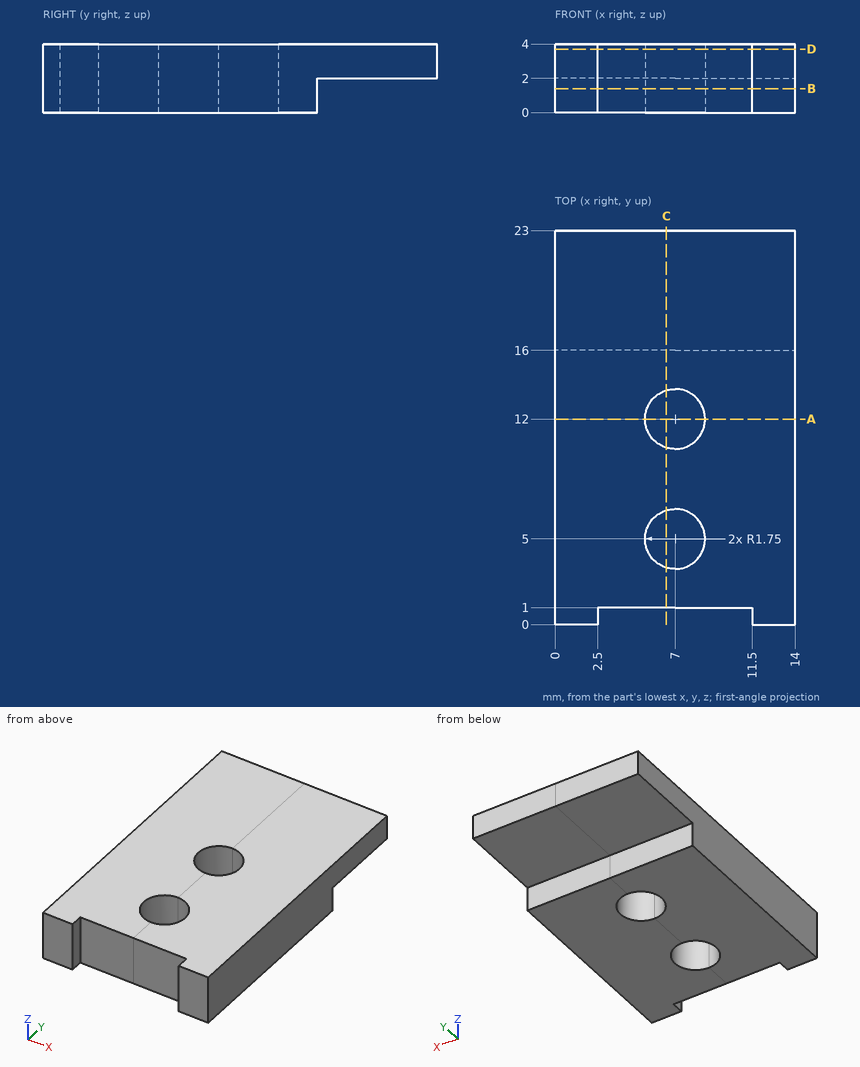
Here's the drawing with two shaded views (mm, measured from the low corner). I have some questions. Give positions to 0.01 mm unless a question says otherwise; leave off trailing zeros. Order: outer loops, then holes, each group sorted by start corner. A loop starts at its lowest first (then second) coordinate and runs counter-clockwise, first axis right, second up.
Q1. If I drill on line 1 along X through (y, z) = (12, 2.85); line 2 along Y through (x, z) = (6.75, 1.55); line 3 along Y through (x, z) = (8.25, 1.4), over which ranges is the centre line in solid material (lowest first)?
Q2. I'm going to push flat-ended pins straight in: P1, Ø4, axis at x = 5, y = 16.5, coming from the -Z side; P2, Ø1.2, axis at x = 9.5, z = 3, coming from the -Y side; P3, Ø0.6, axis at x = 4, z = 1, coming from the +Y side; P4, Ø5.5, axis at x = 9.5, y = 19, coming from the -Z side. Where does each tip first touch, or does it pass through?
Q3. Suppose I cut it at A-A, the plane y = 12. Write out the boundary of the cut face in (x, z), and give its area (3 significant figures).
Q4. Suppose I cut it at B-B, the plane z = 1.4. Write out the boundary of the cut face in (x, y).
Q5. Suppose I cut it at D-D, the plane z = 3.7. Write out the boundary of the cut face in (x, y).
Q6. Suppose I cut it at C-C, the plane x = 6.5. Write out the boundary of the cut face in (y, z), and give its area (3 significant figures).
Solution:
1. line 1: x = 0 to 5.25, 8.75 to 14
1. line 2: y = 1 to 3.27, 6.73 to 10.27, 13.73 to 16
1. line 3: y = 1 to 3.78, 6.22 to 10.78, 13.22 to 16
2. P1: stops at z = 0
2. P2: stops at y = 1
2. P3: stops at y = 16
2. P4: stops at z = 2
3. outline: (0, 0) - (5.25, 0) - (5.25, 4) - (0, 4) - close; (8.75, 0) - (14, 0) - (14, 4) - (8.75, 4) - close
3. area: 42.0 mm2
4. outline: (0, 0) - (2.5, 0) - (2.5, 1) - (11.5, 1) - (11.5, 0) - (14, 0) - (14, 16) - (0, 16) - close; hole circle Ø3.5 at (7, 5); hole circle Ø3.5 at (7, 12)
5. outline: (0, 0) - (2.5, 0) - (2.5, 1) - (11.5, 1) - (11.5, 0) - (14, 0) - (14, 23) - (0, 23) - close; hole circle Ø3.5 at (7, 5); hole circle Ø3.5 at (7, 12)
6. outline: (1, 0) - (3.32, 0) - (3.32, 4) - (1, 4) - close; (6.68, 0) - (10.32, 0) - (10.32, 4) - (6.68, 4) - close; (13.68, 0) - (16, 0) - (16, 2) - (23, 2) - (23, 4) - (13.68, 4) - close
6. area: 47.2 mm2
